```python
from build123d import *

# Parameters (mm, degrees)
SKETCH2_W           = 24.13
SKETCH2_H           = 12.7
SKETCH2_R           = 2.413
BOSS_EXTRUDE1_DEPTH = 8.255
SKETCH3_W           = 1.016
SKETCH3_H           = 12.7
BOSS_EXTRUDE2_DEPTH = 6.35
SKETCH4_R           = 6.985
CUT_EXTRUDE1_DEPTH  = 4.572
SKETCH5_W           = 1.016
SKETCH5_H           = 12.7
BOSS_EXTRUDE3_DEPTH = 6.35


with BuildPart() as part:
    # Sketch2 → Boss-Extrude1 (new body)
    with BuildSketch(Plane(origin=(0, 0, 0), x_dir=(1, 0, 0), z_dir=(0, 1, 0))):
        with Locations((12.223927374, 7.715072626)):
            Rectangle(SKETCH2_W, SKETCH2_H)
        with Locations(Location((12.223927374, 7.715072626, 0), (0, 0, 270))):  # turned: the seam where the file's is
            Circle(SKETCH2_R, mode=Mode.SUBTRACT)
    extrude(amount=BOSS_EXTRUDE1_DEPTH)

    # Sketch3 → Boss-Extrude2 (add)
    with BuildSketch(Plane(origin=(0, 8.255, 0), x_dir=(1, 0, 0), z_dir=(0, 1, 0))):
        with Locations((0.666927374, 7.715072626)):
            Rectangle(SKETCH3_W, SKETCH3_H)
    extrude(amount=BOSS_EXTRUDE2_DEPTH)

    # Sketch4 → Cut-Extrude1 (cut)
    with BuildSketch(Plane.XZ):
        with Locations((12.223927374, -7.715072626)):
            Circle(SKETCH4_R)
    extrude(amount=-CUT_EXTRUDE1_DEPTH, mode=Mode.SUBTRACT)

    # Sketch5 → Boss-Extrude3 (add)
    with BuildSketch(Plane(origin=(0, 8.255, 0), x_dir=(1, 0, 0), z_dir=(0, 1, 0))):
        with Locations((23.780927374, 7.715072626)):
            Rectangle(SKETCH5_W, SKETCH5_H)
    extrude(amount=BOSS_EXTRUDE3_DEPTH)


solid = part.part
```
The listing builds one solid part. Answer for the finished solid, in the listing's coordinates (mm). A direction names the side the tool comes from. Give positions to 0.01 mm unless a question says otherwise; leave off trailing zeros. Order: outer loops, then holes, each group sorted by start corner. A loop starts at its lowest first (then second) coordinate and runs counter-clockwise, first axis right, second up. Notation, with made-up numbers: (29, 65.25) - (39, 65.25) arc R9 cw to (39, 81.25) - close; hole circle Ø9 at (88.25, -5). An arc over 180 degrees is marked (long way). Use one line per item in the form item = value. Start each with the question number.
(1) The mould has two halves that part along Z. Classify faces 4 (the flat face through (4, 0, -8)), 5 (the cylindrical face through (19.208, 2.254, -7.827)), 6 (the flat face through (12, 6, -1.365)), 7 (the cylindrical face through (5.24, 2.25, -7.6)): released by +Z, released by -Z, zero draft, split by the parting line, or undercut.
(2) A cutting plane is placed at A-A, the plane y = 11.5. Write down the section's boundary in (x, z), then the cut area to 3 significant figures.
(3) Consider line 1 (X direction, y = 10.75, z = -3.5); line 2 (X direction, y = 8, z = -7.75); line 3 (Y direction, x = 2.5, z = -10.75) (3 decimals). Determine where each line is inside the solid, lowest interval first. Write a range as from..to.
(4) A cutting plane is placed at B-B, the plane x = 10.5. Write down the section's boundary in (y, z) (3 decimals).
(5) A cutting plane is placed at C-C, the plane z = -7.25. Write down the section's boundary in (x, y) (3 decimals).
(6) For faces 1 (the flat face through (12, 4.572, -5)), 2 (the flat face through (9.6, 8.255, -7.8)), 3 (the flat face through (1, 14.605, -8)), determine the directions among +Z, -Z, +X, -X, +Y, -Y from which every point of the face is accessible in a straight line to the end or side of a thin tool.
(7) Flat-ended cylindrical pins translate along their axes: pin 1 Ø4 at (x, z) = (10, -10.5) entering from -Y; pin 2 Ø4 at (x, z) = (14, -5) entering from +Y (3 decimals). Find the tip coordinate at first contact, or state that the pin passes through.
(8) A cutting plane is placed at D-D, the plane z = -11. Write down the section's boundary in (x, y) (3 decimals), then the cut area to 3 significant figures.
Ans:
q1.face_4 = zero draft
q1.face_5 = undercut
q1.face_6 = released by +Z
q1.face_7 = undercut
q2.outline = (0.16, -14.07) - (1.17, -14.07) - (1.17, -1.37) - (0.16, -1.37) - close; (23.27, -14.07) - (24.29, -14.07) - (24.29, -1.37) - (23.27, -1.37) - close
q2.area = 25.8 mm^2
q3.line_1 = 0.16..1.17, 23.27..24.29
q3.line_2 = 0.16..9.81, 14.64..24.29
q3.line_3 = 0..8.255
q4.outline = (4.572, -14.065) - (8.255, -14.065) - (8.255, -9.403) - (4.572, -9.403) - close; (4.572, -6.027) - (8.255, -6.027) - (8.255, -1.365) - (4.572, -1.365) - close
q5.outline = (0.159, 0) - (5.254, 0) - (5.254, 4.572) - (9.856, 4.572) - (9.856, 8.255) - (1.175, 8.255) - (1.175, 14.605) - (0.159, 14.605) - close; (14.592, 4.572) - (19.193, 4.572) - (19.193, 0) - (24.289, 0) - (24.289, 14.605) - (23.273, 14.605) - (23.273, 8.255) - (14.592, 8.255) - close
q6.face_1 = -Y
q6.face_2 = +Z, -Z, +Y
q6.face_3 = +Z, -Z, +X, -X, +Y
q7.pin_1 = 4.57
q7.pin_2 = 8.255
q8.outline = (0.159, 0) - (6.06, 0) - (6.06, 4.572) - (18.388, 4.572) - (18.388, 0) - (24.289, 0) - (24.289, 14.605) - (23.273, 14.605) - (23.273, 8.255) - (1.175, 8.255) - (1.175, 14.605) - (0.159, 14.605) - close
q8.area = 156 mm^2
